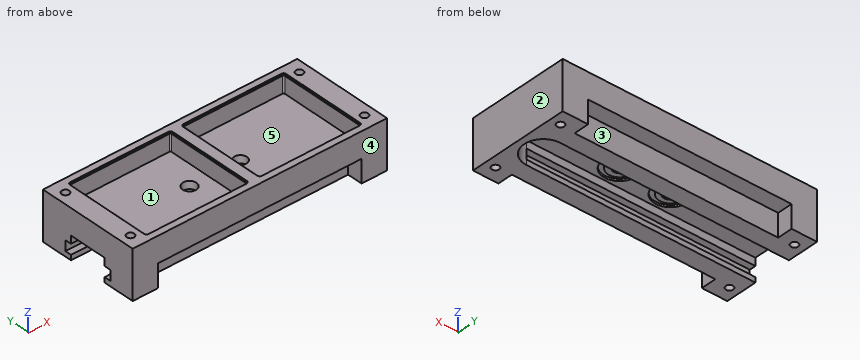
```python
from build123d import *

# Parameters (mm, degrees)
SKETCH1_W           = 100
SKETCH1_H           = 40
BOSS_EXTRUDE1_DEPTH = 38
CUT_EXTRUDE2_START  = -12
SKETCH2_W           = 39.5
SKETCH2_H           = 34
CUT_EXTRUDE2_DEPTH  = 21
CUT_EXTRUDE4_REACH  = 81.36
SKETCH4_R           = 1.45
SKETCH6_W           = 100
SKETCH6_H           = 19
CUT_EXTRUDE5_DEPTH  = 87.215210375
FILLET1_R           = 0.5
CUT_EXTRUDE6_START  = 6.5
CUT_EXTRUDE6_DEPTH  = 0.5
CUT_EXTRUDE6_TAPER  = 2
CUT_EXTRUDE7_START  = 6.5
CUT_EXTRUDE7_DEPTH  = 0.5
CUT_EXTRUDE7_TAPER  = 2
CUT_EXTRUDE12_DEPTH = 9
CUT_EXTRUDE13_REACH = 72.385
SKETCH18_R          = 2.506862912
SKETCH18_R_2        = 2.693115416
SKETCH19_R          = 6.477
SKETCH19_R_2        = 4.572
CUT_EXTRUDE14_DEPTH = 0.79375
SKETCH21_W          = 10
SKETCH21_H          = 15
CUT_EXTRUDE15_DEPTH = 9
SKETCH22_W          = 4
SKETCH22_H          = 2.5
CUT_EXTRUDE16_DEPTH = 90
SKETCH23_W          = 80
SKETCH23_H          = 6
CUT_EXTRUDE17_DEPTH = 9


with BuildPart() as part:
    # Sketch1 → Boss-Extrude1 (new body)
    with BuildSketch(Plane.XY):
        with Locations((16.25, 1.5625)):
            Rectangle(SKETCH1_W, SKETCH1_H)
    extrude(amount=BOSS_EXTRUDE1_DEPTH)

    # Sketch2 → Cut-Extrude2 (cut)
    with BuildSketch(Plane(origin=(0, 0, 0), x_dir=(-1, 0, 0), z_dir=(0, 0, -1)).offset(CUT_EXTRUDE2_START)):
        with Locations((-38.5, 1.5625)):
            Rectangle(SKETCH2_W, SKETCH2_H)
        with Locations((6, 1.5625)):
            Rectangle(SKETCH2_W, SKETCH2_H)
    extrude(amount=-CUT_EXTRUDE2_DEPTH, mode=Mode.SUBTRACT)

    # Sketch4 → Cut-Extrude4 (cut, up to next)
    with BuildSketch(Plane(origin=(0, 0, 0), x_dir=(-1, 0, 0), z_dir=(0, 0, -1)), mode=Mode.PRIVATE) as cut_extrude4_sk1:
        with Locations((-62.25, 16.0625)):
            Circle(SKETCH4_R)
    cut_extrude4_tool1 = extrude(cut_extrude4_sk1.sketch, amount=-CUT_EXTRUDE4_REACH, mode=Mode.PRIVATE) & part.part
    # Sketch4 → Cut-Extrude4 (cut, up to next)
    with BuildSketch(Plane(origin=(0, 0, 0), x_dir=(-1, 0, 0), z_dir=(0, 0, -1)), mode=Mode.PRIVATE) as cut_extrude4_sk2:
        with Locations((-62.25, -12.9375)):
            Circle(SKETCH4_R)
    cut_extrude4_tool2 = extrude(cut_extrude4_sk2.sketch, amount=-CUT_EXTRUDE4_REACH, mode=Mode.PRIVATE) & part.part
    # Sketch4 → Cut-Extrude4 (cut, up to next)
    with BuildSketch(Plane(origin=(0, 0, 0), x_dir=(-1, 0, 0), z_dir=(0, 0, -1)), mode=Mode.PRIVATE) as cut_extrude4_sk3:
        with Locations((29.75, 16.0625)):
            Circle(SKETCH4_R)
    cut_extrude4_tool3 = extrude(cut_extrude4_sk3.sketch, amount=-CUT_EXTRUDE4_REACH, mode=Mode.PRIVATE) & part.part
    # Sketch4 → Cut-Extrude4 (cut, up to next)
    with BuildSketch(Plane(origin=(0, 0, 0), x_dir=(-1, 0, 0), z_dir=(0, 0, -1)), mode=Mode.PRIVATE) as cut_extrude4_sk4:
        with Locations((29.75, -12.9375)):
            Circle(SKETCH4_R)
    cut_extrude4_tool4 = extrude(cut_extrude4_sk4.sketch, amount=-CUT_EXTRUDE4_REACH, mode=Mode.PRIVATE) & part.part
    add(cut_extrude4_tool1.solids().sort_by_distance((62.25, 16.0625, 0))[0], mode=Mode.SUBTRACT)
    add(cut_extrude4_tool2.solids().sort_by_distance((62.25, -12.9375, 0))[0], mode=Mode.SUBTRACT)
    add(cut_extrude4_tool3.solids().sort_by_distance((-29.75, 16.0625, 0))[0], mode=Mode.SUBTRACT)
    add(cut_extrude4_tool4.solids().sort_by_distance((-29.75, -12.9375, 0))[0], mode=Mode.SUBTRACT)

    # Sketch6 → Cut-Extrude5 (cut, through all)
    with BuildSketch(Plane(origin=(0, 21.5625, 0), x_dir=(1, 0, 0), z_dir=(0, 1, 0))):
        with Locations((16.25, -28.5)):
            Rectangle(SKETCH6_W, SKETCH6_H)
    extrude(amount=-CUT_EXTRUDE5_DEPTH, mode=Mode.SUBTRACT)

    # Fillet1
    fillet1_edges = [part.edges().sort_by_distance(p)[0] for p in [
        (-25.75, -15.4375, 15.5),
        (13.75, -15.4375, 15.5),
        (-25.75, 18.5625, 15.5),
        (13.75, 18.5625, 15.5),
        (18.75, -15.4375, 15.5),
        (58.25, -15.4375, 15.5),
        (18.75, 18.5625, 15.5),
        (58.25, 18.5625, 15.5),
    ]]
    fillet(fillet1_edges, radius=FILLET1_R)

    # Sketch10 → Cut-Extrude6 (cut)
    with BuildSketch(Plane.XY.offset(12).offset(CUT_EXTRUDE6_START)):
        with BuildLine():
            Line((14.25, -14.9375), (14.25, 18.0625))
            ThreePointArc((14.25, 18.0625), (13.957106781, 18.769606781), (13.25, 19.0625))
            Line((13.25, 19.0625), (-25.25, 19.0625))
            ThreePointArc((-25.25, 19.0625), (-25.957106781, 18.769606781), (-26.25, 18.0625))
            Line((-26.25, 18.0625), (-26.25, -14.9375))
            ThreePointArc((-26.25, -14.9375), (-25.957106781, -15.644606781), (-25.25, -15.9375))
            Line((-25.25, -15.9375), (13.25, -15.9375))
            ThreePointArc((13.25, -15.9375), (13.957106781, -15.644606781), (14.25, -14.9375))
        make_face()
    extrude(amount=CUT_EXTRUDE6_DEPTH, taper=CUT_EXTRUDE6_TAPER, mode=Mode.SUBTRACT)

    # Sketch11 → Cut-Extrude7 (cut)
    with BuildSketch(Plane.XY.offset(12).offset(CUT_EXTRUDE7_START)):
        with BuildLine():
            Line((58.75, -14.9375), (58.75, 18.0625))
            ThreePointArc((58.75, 18.0625), (58.457106781, 18.769606781), (57.75, 19.0625))
            Line((57.75, 19.0625), (19.25, 19.0625))
            ThreePointArc((19.25, 19.0625), (18.542893219, 18.769606781), (18.25, 18.0625))
            Line((18.25, 18.0625), (18.25, -14.9375))
            ThreePointArc((18.25, -14.9375), (18.542893219, -15.644606781), (19.25, -15.9375))
            Line((19.25, -15.9375), (57.75, -15.9375))
            ThreePointArc((57.75, -15.9375), (58.457106781, -15.644606781), (58.75, -14.9375))
        make_face()
    extrude(amount=CUT_EXTRUDE7_DEPTH, taper=CUT_EXTRUDE7_TAPER, mode=Mode.SUBTRACT)

    # Sketch17 → Cut-Extrude12 (cut)
    with BuildSketch(Plane(origin=(0, 0, 0), x_dir=(-1, 0, 0), z_dir=(0, 0, -1))):
        with BuildLine():
            Line((-56.25, 9.0625), (23.75, 9.0625))
            ThreePointArc((23.75, 9.0625), (31.25, 1.5625), (23.75, -5.9375))
            Line((23.75, -5.9375), (-56.25, -5.9375))
            ThreePointArc((-56.25, -5.9375), (-63.75, 1.5625), (-56.25, 9.0625))
        make_face()
    extrude(amount=-CUT_EXTRUDE12_DEPTH, mode=Mode.SUBTRACT)

    # Sketch18 → Cut-Extrude13 (cut, up to next)
    with BuildSketch(Plane(origin=(0, 0, 9), x_dir=(-1, 0, 0), z_dir=(0, 0, -1)), mode=Mode.PRIVATE) as cut_extrude13_sk1:
        with Locations((-26.25, 1.5625)):
            Circle(SKETCH18_R)
    cut_extrude13_tool1 = extrude(cut_extrude13_sk1.sketch, amount=-CUT_EXTRUDE13_REACH, mode=Mode.PRIVATE) & part.part
    # Sketch18 → Cut-Extrude13 (cut, up to next)
    with BuildSketch(Plane(origin=(0, 0, 9), x_dir=(-1, 0, 0), z_dir=(0, 0, -1)), mode=Mode.PRIVATE) as cut_extrude13_sk2:
        with Locations((-6.25, 1.5625)):
            Circle(SKETCH18_R_2)
    cut_extrude13_tool2 = extrude(cut_extrude13_sk2.sketch, amount=-CUT_EXTRUDE13_REACH, mode=Mode.PRIVATE) & part.part
    add(cut_extrude13_tool1.solids().sort_by_distance((26.25, 1.5625, 9))[0], mode=Mode.SUBTRACT)
    add(cut_extrude13_tool2.solids().sort_by_distance((6.25, 1.5625, 9))[0], mode=Mode.SUBTRACT)

    # Sketch19 → Cut-Extrude14 (cut)
    # profile 1 of 2: a face of its own
    with BuildSketch(Plane(origin=(0, 0, 9), x_dir=(-1, 0, 0), z_dir=(0, 0, -1))):
        with Locations((-26.25, 1.5625)):
            Circle(SKETCH19_R)
        with Locations((-26.25, 1.5625)):
            Circle(SKETCH19_R_2, mode=Mode.SUBTRACT)
    # profile 2 of 2: a face of its own
    with BuildSketch(Plane(origin=(0, 0, 9), x_dir=(-1, 0, 0), z_dir=(0, 0, -1))):
        with Locations((-6.25, 1.5625)):
            Circle(SKETCH19_R)
        with Locations((-6.25, 1.5625)):
            Circle(SKETCH19_R_2, mode=Mode.SUBTRACT)
    extrude(amount=-CUT_EXTRUDE14_DEPTH, mode=Mode.SUBTRACT)

    # Sketch21 → Cut-Extrude15 (cut)
    with BuildSketch(Plane(origin=(0, 0, 0), x_dir=(-1, 0, 0), z_dir=(0, 0, -1))):
        with Locations((28.75, 1.5625)):
            Rectangle(SKETCH21_W, SKETCH21_H)
    extrude(amount=-CUT_EXTRUDE15_DEPTH, mode=Mode.SUBTRACT)

    # Sketch22 → Cut-Extrude16 (cut)
    with BuildSketch(Plane.ZY.offset(33.75)):
        with Locations((4, 10.3125)):
            Rectangle(SKETCH22_W, SKETCH22_H)
        with Locations((4, -7.1875)):
            Rectangle(SKETCH22_W, SKETCH22_H)
    extrude(amount=-CUT_EXTRUDE16_DEPTH, mode=Mode.SUBTRACT)

    # Sketch23 → Cut-Extrude17 (cut)
    with BuildSketch(Plane(origin=(0, 0, 0), x_dir=(-1, 0, 0), z_dir=(0, 0, -1))):
        with Locations((-16.25, 18.5625)):
            Rectangle(SKETCH23_W, SKETCH23_H)
        with Locations((-16.25, -15.4375)):
            Rectangle(SKETCH23_W, SKETCH23_H)
    extrude(amount=-CUT_EXTRUDE17_DEPTH, mode=Mode.SUBTRACT)


solid = part.part
```
Verification items for the finished model (mm, model axes). Face numbers are marked on the shaded views. A direction names the side the tool comes from. Coordinates: 2 decimals unless noted, no trailing zeros. Write each loop counter-clockwise with the first axis right and the second up, starting at its lowest first coordinate (ties: lowest second). Pieces come first, ordered by that corner, then holes. Notation, with made-up numbers: M 33,43 L 66,43 A31 ccw 66,67 Z; hole C -9.5,58 d1. An arc over 180 degrees is marked long. Answer as a JSON object with one key per item and string values. Group by question number.
(1) Material ranges on line 1 (Y direction, x = 6.25, z = 9.65); line 2 (X direction, y = -0.5, z = 16); line 3 (X direction, y = 17, z = 4.5), recorded low to high.
(2) Tool access check on the marked faces 1 and 2. Record the directions out of +Z, -Z, +X, -X, +Y, -Y that give a thin tool (end or side, any length) a straight path to the whole face; none if there is none.
(3) Cross-section at C-C, the plane z = 17.5. Record the cut outline in (x, y), and give its area (3 significant figures).
(4) Cross-section at A-A, the plane x = -29.75. Record the cut outline in (y, z), and give its area (3 significant figures).
(5) Cross-section at B-B, the plane x = 42. Record the cut outline in (y, z).
(6) Gauge pin test, flat ends, axial feed: pin 1 (1.5 mm diameter, centred on x = -3, z = 7, fed in from -Y); pin 2 (3 mm diameter, centred on x = -19, y = 0, fed in from -Z); pin 3 (5 mm diameter, centred on x = -9, y = 12, fed in from +Z); pin 4 (3 mm diameter, centred on x = 54, y = -10, fed in from -Z). Record the tip position at first contact, or that the pin passes through.
(7) Release check for a two-part mould opening along Y. For the marked faces 3, 4 and 5 record: +Y half, -Y half, draft (parallel to the pull), parting line (faces both ways), or undercut.
(8) Cross-section at D-D, the plane x = 62.25. Record the cut outline in (y, z).
Reply:
{
 "1": {"line 1": "-18.44 to -4.91, -3.01 to -1.13, 4.26 to 6.13, 8.04 to 21.56", "line 2": "-33.75 to -25.75, 13.75 to 18.75, 58.25 to 66.25", "line 3": "-33.75 to -30.86, -28.64 to -23.75, 56.25 to 61.14, 63.36 to 66.25"},
 "2": {"face 1": "+Z", "face 2": "+Z, -Z, +X, +Y, -Y"},
 "3": {"outline": "M -33.75,-18.44 L 66.25,-18.44 L 66.25,21.56 L -33.75,21.56 Z; hole C -29.75,-12.94 d2.9; hole C -29.75,16.06 d2.9; hole M -25.75,-14.94 A0.5 ccw -25.25,-15.44 L 13.25,-15.44 A0.5 ccw 13.75,-14.94 L 13.75,18.06 A0.5 ccw 13.25,18.56 L -25.25,18.56 A0.5 ccw -25.75,18.06 Z; hole M 18.75,-14.94 A0.5 ccw 19.25,-15.44 L 57.75,-15.44 A0.5 ccw 58.25,-14.94 L 58.25,18.06 A0.5 ccw 57.75,18.56 L 19.25,18.56 A0.5 ccw 18.75,18.06 Z; hole C 62.25,-12.94 d2.9; hole C 62.25,16.06 d2.9", "area": "1,290 mm²"},
 "4": {"outline": "M -18.44,0 L -14.39,0 L -14.39,19 L -18.44,19 Z; M -11.49,0 L -5.94,0 L -5.94,2 L -8.44,2 L -8.44,6 L -5.94,6 L -5.94,9 L 9.06,9 L 9.06,6 L 11.56,6 L 11.56,2 L 9.06,2 L 9.06,0 L 14.61,0 L 14.61,19 L -11.49,19 Z; M 17.51,0 L 21.56,0 L 21.56,19 L 17.51,19 Z", "area": "495 mm²"},
 "5": {"outline": "M -18.44,9 L -12.44,9 L -12.44,0 L -5.94,0 L -5.94,2 L -8.44,2 L -8.44,6 L -5.94,6 L -5.94,9 L 9.06,9 L 9.06,6 L 11.56,6 L 11.56,2 L 9.06,2 L 9.06,0 L 15.56,0 L 15.56,9 L 21.56,9 L 21.56,19 L 19.05,19 L 19.06,18.5 L 18.56,18.5 L 18.56,12 L -15.44,12 L -15.44,18.5 L -15.94,18.5 L -15.92,19 L -18.44,19 Z"},
 "6": {"pin 1": "y = -12.44", "pin 2": "z = 9", "pin 3": "z = 12", "pin 4": "z = 0"},
 "7": {"face 3": "+Y half", "face 4": "-Y half", "face 5": "undercut"},
 "8": {"outline": "M -18.44,0 L -14.39,0 L -14.39,19 L -18.44,19 Z; M -11.49,0 L -2.94,0 L -2.94,9 L 6.06,9 L 6.06,0 L 14.61,0 L 14.61,19 L -11.49,19 Z; M 17.51,0 L 21.56,0 L 21.56,19 L 17.51,19 Z"}
}
